Autodesk Fusion 360 part; units mm, degrees
sketch "Sketch1" plane through (0, 0, 0) normal (1, 0, 0) x (0, 0, -1)
  line L0 (17.3205, -30) -> (34.641, 0)
  line L1 (34.641, 0) -> (17.3205, 30)
  line L2 (17.3205, 30) -> (-17.3205, 30)
  line L3 (-17.3205, 30) -> (-34.641, 0)
  line L4 (-34.641, 0) -> (-17.3205, -30)
  line L5 (-17.3205, -30) -> (17.3205, -30)
  line L6 (-17.3205, 30) -> (2.6795, 30) construction
  line L7 (2.6795, 30) -> (2.6795, -30) construction
  line L8 (2.6795, -30) -> (-17.3205, -30) construction
  line L9 (-17.3205, -30) -> (-17.3205, 30) construction
  line L10 (-17.3205, 0) -> (2.6795, 0)
  line L11 (-17.3205, 30) -> (-17.3205, 0)
  line L12 (-17.3205, 0) -> (-17.3205, -30)
  line L13 (-17.3205, 0) -> (2.6795, -30) construction
  line L14 (-17.3205, 0) -> (2.6795, 30) construction
  circle A0 centre (-7.3205, 15) radius 1.7
  circle A1 centre (-7.3205, -15) radius 1.7
  circle A2 centre (-7.3205, 15) radius 3
  circle A3 centre (-7.3205, -15) radius 3
  line L15 (-7.3205, 30) -> (-7.3205, -30) construction
  line L16 (-4.4205, 25) -> (-10.2205, 25)
  line L17 (-10.2205, 25) -> (-10.2205, 35)
  line L18 (-10.2205, 35) -> (-4.4205, 35)
  line L19 (-4.4205, 35) -> (-4.4205, 25)
  line L20 (-4.4205, 25) -> (-10.2205, 35) construction
  line L21 (-10.2205, 25) -> (-4.4205, 35) construction
  line L22 (-4.4205, -35) -> (-10.2205, -35)
  line L23 (-10.2205, -35) -> (-10.2205, -25)
  line L24 (-10.2205, -25) -> (-4.4205, -25)
  line L25 (-4.4205, -25) -> (-4.4205, -35)
  line L26 (-4.4205, -35) -> (-10.2205, -25) construction
  line L27 (-10.2205, -35) -> (-4.4205, -25) construction
  line L28 (-17.3205, 30) -> (-17.3205, -30)
  line L29 (-17.3205, -30) -> (-21.5905, -30)
  line L30 (-21.5905, -30) -> (-21.5905, 30)
  line L31 (-21.5905, 30) -> (-17.3205, 30)
  line L32 (30, -17.3205) -> (30, 17.3205)
  line L33 (30, 17.3205) -> (0, 34.641)
  line L34 (0, 34.641) -> (-30, 17.3205)
  line L35 (-30, 17.3205) -> (-30, -17.3205)
  line L36 (-30, -17.3205) -> (0, -34.641)
  line L37 (0, -34.641) -> (30, -17.3205)
  point P0 (-7.3205, 30)
  point P1 (-7.3205, -30)
  dimension "d1" = 30
  dimension "d2" = 20
  dimension "d3" = 3.4
  dimension "d4" = 3.4
  dimension "d5" = 6
  dimension "d6" = 6
  dimension "d7" = 5.8
  dimension "d8" = 10
  dimension "d9" = 5.8
  dimension "d10" = 10
  dimension "d11" = 4.27
  dimension "d12" = 30
extrude "Extrude1" add sketch "Sketch1" along normal blind 6 contours L0 L1 L2 L5 L11 L12 L16 L17 L19 L23 L24 L25 L28 L32 L33 L34 L36 L37 | L0 L32 L37 | L5 L25 L36 L37 | L5 L25 L36 | L5 L23 L24 L25 L36 | L1 L32 L33 | L2 L19 L33 L34 | L2 L16 L17 L19 L34 | L2 L19 L34
extrude "Extrude2" add sketch "Sketch1" against normal blind 5 contours L5 L25 L36 | L5 L23 L24 L25 L36 | L2 L16 L17 L19 L34 | L2 L19 L34
extrude "Extrude3" add sketch "Sketch1" along normal blind 3 contours A2 | A3
fillet "Fillet1" radius 3.25 6 edges at (3, -34.641, 0) (3, -17.3205, -30) (3, 17.3205, -30) (3, 34.641, 0) (3, 24.641, 17.3205) (3, -24.641, 17.3205)
chamfer "Chamfer1" distance 2 angle 45 12 edges at (6, -25.9808, -15) (6, -17.0691, -29.5646) (6, 0, -30) (6, 17.0691, -29.5646) (6, 25.9808, -15) (6, 34.1382, 0) (6, 29.641, 8.6603) (6, 24.3896, 16.8851) (6, 0, 17.3205) (6, -24.3896, 16.8851) (6, -29.641, 8.6603) (6, -34.1382, 0)
fillet "Fillet2" radius 1 9 edges at (-2.5, 25, 4.4205) (-2.5, 25, 10.2205) (-2.5, -32.0888, 4.4205) (-2.5, -28.7402, 10.2205) (-2.5, -25, 10.2205) (-2.5, -25, 4.4205) (-5, -25, 7.3205) (-2.5, 28.7402, 10.2205) (-2.5, 32.0888, 4.4205) 2 faces at (-5, -28.6097, 6.3538) (-5, 28.6097, 6.3538)
Build history of the part. All positions in model axes, mm. A direction names the side the tool comes from. Coordinates: 2 decimals unless noted, no trailing zeros. Write each loop counter-clockwise with the first axis right and the second up, starting at its lowest first coordinate (ties: lowest second). Pieces come first, ordered by that corner, then holes. Notation, with made-up numbers: (-10, 1.25) -> (32, 1.25) arc R8 cw to (32, 5.25) -> close; hole circle Ø1 at (-37, -15.75). An arc over 180 degrees is marked (long way). Use CSV: the item, a comma, the result in double quotes. Start each with the question number.
Q1. Drill centre lines: probe 1 along X at (y, z) = (-13.5, -25); probe 2 along X at (y, z) = (17, 9); probe 3 along Y at (x, z) = (4.25, -8.5). Where is each one in solid material? Low to high.
Q2. Cut at D-D, the plane z = -21. List the corners of the cut face in (x, y).
Q3. Cut at A-A, the plane x = -1.5. List the corners of the cut face in (y, z), then the cut area to 3 significant figures.
Q4. 3-axis set-ups, long thin cutter, end or side, ignore diameter. For faces 5 (the flat face through (-2, -28, 4.42)), 6 (the flat face through (-2, -25, 7)), 7 (the flat face through (-2, 27, 10.22)): which of +Z, -Z, +X, -X, +Y, -Y reach the whole face in a straight line?
Q5. Pull direction Z, two halves, no side cores. Call faces 1 (the flat face through (1.722, -29.584, 8.759)), 2 (the cylindrical face through (2.03, 34.14, -0.02)), 3 (the cylindrical face through (1.48, 14.93, 9.02)), 4 (the conical face through (4.986, -16.562, -28.719)): released by +Z, released by -Z, zero draft, split by the parting line, or undercut.
Q6. Flat gauge pins, fed straight in: pin 1 Ø2 at (x, z) = (3.5, 10.5) entering from +Y; pin 2 Ø5.5 at (y, z) = (15, 7.32) entering from +X; pin 3 Ø0.6 at (x, y) = (-2.5, 27) entering from +Z. Where does each tip first touch, or does it go through?
Q7. Cut at B-B, the plane x = 5. State how many separate pieces and enclosed holes the cut face has, then the cut area to 3 significant figures.
Q8. Cut at C-C, the plane y = -27. List the corners of the cut face in (x, z).
Checked values:
1,probe 1,"x = 0 to 6"
1,probe 2,"x = 0 to 3"
1,probe 3,"y = -29.44 to 29.44"
2,outline,"(0, -22.52) -> (4, -22.52) -> (6, -20.21) -> (6, 20.21) -> (4, 22.52) -> (0, 22.52) -> close"
3,outline,"(-31.22, 5.92) arc R1 ccw to (-30.36, 4.42) -> (-26, 4.42) arc R1 ccw to (-25, 5.42) -> (-25, 9.22) arc R1 ccw to (-26, 10.22) -> (-28.16, 10.22) arc R1 ccw to (-29.03, 9.72) -> close; (25, 5.42) arc R1 ccw to (26, 4.42) -> (30.36, 4.42) arc R1 ccw to (31.22, 5.92) -> (29.03, 9.72) arc R1 ccw to (28.16, 10.22) -> (26, 10.22) arc R1 ccw to (25, 9.22) -> close"
3,area,"60.5 mm²"
4,face 5,"-Z, -X, +Y, -Y"
4,face 6,"+Z, -Z, -X"
4,face 7,"+Z, -X, +Y, -Y"
5,face 1,"released by +Z"
5,face 2,"split by the parting line"
5,face 3,"undercut"
5,face 4,"released by -Z"
6,pin 1,"stops at y = 29.16"
6,pin 2,"stops at x = 3"
6,pin 3,"stops at z = 10.22"
7,separate pieces,"1"
7,enclosed holes,"2"
7,area,"2,340 mm²"
8,outline,"(-5, 5.42) arc R1 ccw to (-4, 4.42) -> (0, 4.42) -> (0, -13.23) -> (4, -13.23) -> (6, -9.23) -> (6, 9.23) -> (4, 13.23) -> (0, 13.23) -> (0, 10.22) -> (-4, 10.22) arc R1 ccw to (-5, 9.22) -> close"
